The model under review builds one solid part; all positions refer to its coordinate system, in mm. Face numbers are marked on the shaded views. A direction names the side the tool comes from. Round coordinates to 2 decimals unless told otherwise and drop trailing zeros. Order: outer loops, then holes, each group sorted by start corner. A loop starts at its lowest first (then second) coordinate and runs counter-clockwise, first axis right, second up.
1) Clearance check with flat-ended pins moving along their axes: P1, Ø4, axis at y = 148.5, z = 55.5, coming from the -X side; P2, Ø9.5, axis at x = 0, y = 0, coming from the -Z side; P3, Ø3, axis at x = -1.5, y = -15, coming from the -Z side. State where each tip first meets the part, or that it passes through.
2) Mouldability with a two-part tool opening along Z and no side actions: class the marked faces 6, 7 and 8 as pulls with the +Z half, pulls with the -Z half, needs draft (parallel to the pull), parting line crosses it, or undercut.
3) Consider section B-B (y = 62.5). Give the boundary of the cut face in (x, z), then the cut area to 3 significant figures.
4) Machinability: for the marked faces 1, 2, 3, 4 and 5, which of the approach directions +Z, -Z, +X, -X, +Y, -Y give a long, thin tool a straight path to every point of the face, cutting with its end or side? Answer none if there is none.
5) To check wall thickness, follow L1, parallel to Y at x = 0, z = 11.25; L2, parallel to Z at x = 27, y = -24; L3, parallel to Y at x = 0, z = 4.75 (3 decimals). State the ranges of each line that lie inside material, in increasing order.
6) Consider section C-C (z = 203.5). Give the boundary of the cut face in (x, y), then the cut area to 3 significant figures.
7) Consider section A-A (z = 30.5). Give the boundary of the cut face in (x, y), then the cut area to 3 significant figures.
from build123d import *

# Parameters (mm, degrees)
SKETCH1_R            = 28.1
BOSS_EXTRUDE2_DEPTH  = 24
CUT_EXTRUDE2_DEPTH   = 21.5
SKETCH4_R            = 3
CUT_EXTRUDE3_DEPTH   = 9.5
SKETCH6_R            = 6.025
CUT_EXTRUDE4_DEPTH   = 6.2
SKETCH7_W            = 56.2
SKETCH7_H            = 56.2
BOSS_EXTRUDE3_DEPTH  = 56.2
SKETCH8_W            = 56.2
SKETCH8_H            = 56.2
BOSS_EXTRUDE4_DEPTH  = 14.14
SKETCH10_W           = 56.2
SKETCH10_H           = 56.2
BOSS_EXTRUDE5_DEPTH  = 10
SKETCH11_W           = 10
SKETCH11_H           = 56.2
BOSS_EXTRUDE6_DEPTH  = 146.9
SKETCH12_W           = 10
SKETCH12_H           = 56.2
BOSS_EXTRUDE7_DEPTH  = 126.9
SKETCH13_W           = 10
SKETCH13_H           = 56.2
BOSS_EXTRUDE8_DEPTH  = 146.9
SKETCH14_W           = 10
SKETCH14_H           = 56.2
BOSS_EXTRUDE9_DEPTH  = 126.9
SKETCH15_W           = 10
SKETCH15_H           = 56.2
BOSS_EXTRUDE10_DEPTH = 25
SKETCH16_W           = 10
SKETCH16_H           = 56.2
BOSS_EXTRUDE11_DEPTH = 25
SKETCH17_W           = 56.2
SKETCH17_H           = 10
BOSS_EXTRUDE12_DEPTH = 25
SKETCH18_W           = 56.2
SKETCH18_H           = 10
BOSS_EXTRUDE13_DEPTH = 25
SKETCH19_W           = 51.2
SKETCH19_H           = 51.2
CUT_EXTRUDE5_DEPTH   = 63.7
SKETCH23_W           = 330
SKETCH23_H           = 16.2
CUT_EXTRUDE7_DEPTH   = 5
SKETCH24_W           = 16.2
SKETCH24_H           = 290
CUT_EXTRUDE8_DEPTH   = 5
SKETCH25_W           = 16.2
SKETCH25_H           = 16.2
CUT_EXTRUDE12_DEPTH  = 25
CUT_EXTRUDE13_DEPTH  = 56.2
CUT_EXTRUDE14_DEPTH  = 56.2
SKETCH28_W           = 21
SKETCH28_H           = 16.2
CUT_EXTRUDE15_DEPTH  = 5
SKETCH29_W           = 21
SKETCH29_H           = 16.2
CUT_EXTRUDE16_DEPTH  = 5
SKETCH30_W           = 21
SKETCH30_H           = 16.2
CUT_EXTRUDE17_DEPTH  = 5
SKETCH31_W           = 21
SKETCH31_H           = 16.2
CUT_EXTRUDE18_DEPTH  = 5
SKETCH33_R           = 2.65
CUT_EXTRUDE19_DEPTH  = 2.4
SKETCH34_R           = 0.5
CUT_EXTRUDE20_DEPTH  = 10
SKETCH35_R           = 2.65
CUT_EXTRUDE21_DEPTH  = 2.4
SKETCH36_R           = 0.5
CUT_EXTRUDE22_DEPTH  = 10
SKETCH37_R           = 2.65
CUT_EXTRUDE23_DEPTH  = 2.4
SKETCH38_R           = 0.5
CUT_EXTRUDE24_DEPTH  = 10
SKETCH39_R           = 2.65
CUT_EXTRUDE25_DEPTH  = 2.4
SKETCH40_R           = 0.5
CUT_EXTRUDE26_DEPTH  = 10
SKETCH41_R           = 3.75
CUT_EXTRUDE28_DEPTH  = 30


with BuildPart() as part:
    # Sketch1 → Boss-Extrude2 (new body)
    with BuildSketch(Plane.XY):
        Circle(SKETCH1_R)
    extrude(amount=BOSS_EXTRUDE2_DEPTH)

    # Sketch3 → Cut-Extrude2 (cut)
    with BuildSketch(Plane(origin=(0, 0, 0), x_dir=(-1, 0, 0), z_dir=(0, 0, -1))):
        with BuildLine():
            Line((-1.661801922, 2.5), (1.661801922, 2.5))
            ThreePointArc((1.661801922, 2.5), (0, -3.001930317), (-1.661801922, 2.5))
        make_face()
    extrude(amount=-CUT_EXTRUDE2_DEPTH, mode=Mode.SUBTRACT)

    # Sketch4 → Cut-Extrude3 (cut)
    with BuildSketch(Plane(origin=(0, 0, 0), x_dir=(-1, 0, 0), z_dir=(0, 0, -1))):
        Circle(SKETCH4_R)
    extrude(amount=-CUT_EXTRUDE3_DEPTH, mode=Mode.SUBTRACT)

    # Sketch6 → Cut-Extrude4 (cut)
    with BuildSketch(Plane(origin=(0, 0, 0), x_dir=(-1, 0, 0), z_dir=(0, 0, -1))):
        Circle(SKETCH6_R)
    extrude(amount=-CUT_EXTRUDE4_DEPTH, mode=Mode.SUBTRACT)

    # Sketch7 → Boss-Extrude3 (add)
    with BuildSketch(Plane.XY.offset(24)):
        Rectangle(SKETCH7_W, SKETCH7_H)
    extrude(amount=BOSS_EXTRUDE3_DEPTH)

    # Sketch8 → Boss-Extrude4 (add)
    with BuildSketch(Plane(origin=(28.1, 0, 0), x_dir=(0, 0, -1), z_dir=(1, 0, 0))):
        with Locations((-52.1, 0)):
            Rectangle(SKETCH8_W, SKETCH8_H)
    extrude(amount=BOSS_EXTRUDE4_DEPTH)

    # Sketch10 → Boss-Extrude5 (add)
    with BuildSketch(Plane(origin=(42.24, 0, 0), x_dir=(0, 0, -1), z_dir=(1, 0, 0))):
        with Locations((-52.1, 0)):
            Rectangle(SKETCH10_W, SKETCH10_H)
    extrude(amount=BOSS_EXTRUDE5_DEPTH)

    # Sketch11 → Boss-Extrude6 (add)
    with BuildSketch(Plane.XY.offset(80.2)):
        with Locations((47.24, 0)):
            Rectangle(SKETCH11_W, SKETCH11_H)
    extrude(amount=BOSS_EXTRUDE6_DEPTH)

    # Sketch12 → Boss-Extrude7 (add)
    with BuildSketch(Plane(origin=(0, 28.1, 0), x_dir=(1, 0, 0), z_dir=(0, 1, 0))):
        with Locations((47.24, -52.1)):
            Rectangle(SKETCH12_W, SKETCH12_H)
    extrude(amount=BOSS_EXTRUDE7_DEPTH)

    # Sketch13 → Boss-Extrude8 (add)
    with BuildSketch(Plane(origin=(0, 0, 24), x_dir=(-1, 0, 0), z_dir=(0, 0, -1))):
        with Locations((-47.24, 0)):
            Rectangle(SKETCH13_W, SKETCH13_H)
    extrude(amount=BOSS_EXTRUDE8_DEPTH)

    # Sketch14 → Boss-Extrude9 (add)
    with BuildSketch(Plane(origin=(0, -28.1, 0), x_dir=(-1, 0, 0), z_dir=(0, -1, 0))):
        with Locations((-47.24, -52.1)):
            Rectangle(SKETCH14_W, SKETCH14_H)
    extrude(amount=BOSS_EXTRUDE9_DEPTH)

    # Sketch15 → Boss-Extrude10 (add)
    with BuildSketch(Plane(origin=(52.24, 0, 0), x_dir=(0, 0, -1), z_dir=(1, 0, 0))):
        with Locations((-222.1, 0)):
            Rectangle(SKETCH15_W, SKETCH15_H)
    extrude(amount=BOSS_EXTRUDE10_DEPTH)

    # Sketch16 → Boss-Extrude11 (add)
    with BuildSketch(Plane(origin=(52.24, 0, 0), x_dir=(0, 0, -1), z_dir=(1, 0, 0))):
        with Locations((117.9, 0)):
            Rectangle(SKETCH16_W, SKETCH16_H)
    extrude(amount=BOSS_EXTRUDE11_DEPTH)

    # Sketch17 → Boss-Extrude12 (add)
    with BuildSketch(Plane(origin=(52.24, 0, 0), x_dir=(0, 0, -1), z_dir=(1, 0, 0))):
        with Locations((-52.1, 150)):
            Rectangle(SKETCH17_W, SKETCH17_H)
    extrude(amount=BOSS_EXTRUDE12_DEPTH)

    # Sketch18 → Boss-Extrude13 (add)
    with BuildSketch(Plane(origin=(52.24, 0, 0), x_dir=(0, 0, -1), z_dir=(1, 0, 0))):
        with Locations((-52.1, -150)):
            Rectangle(SKETCH18_W, SKETCH18_H)
    extrude(amount=BOSS_EXTRUDE13_DEPTH)

    # Sketch19 → Cut-Extrude5 (cut)
    with BuildSketch(Plane.ZY.offset(28.1)):
        with Locations((52.1, 0)):
            Rectangle(SKETCH19_W, SKETCH19_H)
    extrude(amount=-CUT_EXTRUDE5_DEPTH, mode=Mode.SUBTRACT)

    # Cut-Sweep2: sweep along a path in Sketch20
    with BuildLine(Plane(origin=(0, 0, 0), x_dir=(-1, 0, 0), z_dir=(0, 0, -1))) as cut_sweep2_path:
        ThreePointArc((0, 15), (-10.606601718, 10.606601718), (-15, 0))
    # 3DSketch2 → Cut-Sweep2 (sweep, cut)
    with BuildSketch(Plane(origin=(0, 15, 0), x_dir=(0, 0.17521220324553322, 0.9845306921746249), z_dir=(-1, 0, 0))):
        Polygon((0, 0), (1.314091524, 7.383980191), (42.805237655, 0), (41.491146131, -7.383980191), align=None)
    sweep(path=cut_sweep2_path.line, mode=Mode.SUBTRACT)

    # Sketch23 → Cut-Extrude7 (cut)
    with BuildSketch(Plane(origin=(52.24, 0, 0), x_dir=(0, 0, -1), z_dir=(1, 0, 0))):
        with Locations((-52.1, 0)):
            Rectangle(SKETCH23_W, SKETCH23_H)
    extrude(amount=-CUT_EXTRUDE7_DEPTH, mode=Mode.SUBTRACT)

    # Sketch24 → Cut-Extrude8 (cut)
    with BuildSketch(Plane(origin=(52.24, 0, 0), x_dir=(0, 0, -1), z_dir=(1, 0, 0))):
        with Locations((-52.1, 0)):
            Rectangle(SKETCH24_W, SKETCH24_H)
    extrude(amount=-CUT_EXTRUDE8_DEPTH, mode=Mode.SUBTRACT)

    # Sketch25 → Cut-Extrude12 (cut)
    with BuildSketch(Plane(origin=(47.24, 0, 0), x_dir=(0, 0, -1), z_dir=(1, 0, 0))):
        with Locations((-52.1, 0)):
            Rectangle(SKETCH25_W, SKETCH25_H)
    extrude(amount=-CUT_EXTRUDE12_DEPTH, mode=Mode.SUBTRACT)

    # Sketch26 → Cut-Extrude13 (cut)
    with BuildSketch(Plane(origin=(0, -28.1, 0), x_dir=(-1, 0, 0), z_dir=(0, -1, 0))):
        Polygon((-77.24, -217.1), (-67.24, -227.1), (-77.24, -227.1), align=None)
        Polygon((-77.24, 112.9), (-67.24, 122.9), (-77.24, 122.9), align=None)
    extrude(amount=-CUT_EXTRUDE13_DEPTH, mode=Mode.SUBTRACT)

    # Sketch27 → Cut-Extrude14 (cut)
    with BuildSketch(Plane.XY.offset(80.2)):
        Polygon((77.24, -145), (67.24, -155), (77.24, -155), align=None)
        Polygon((77.24, 145), (67.24, 155), (77.24, 155), align=None)
    extrude(amount=-CUT_EXTRUDE14_DEPTH, mode=Mode.SUBTRACT)

    # Sketch28 → Cut-Extrude15 (cut)
    with BuildSketch(Plane(origin=(0, -145, 0), x_dir=(1, 0, 0), z_dir=(0, 1, 0))):
        with Locations((57.74, -52.1)):
            Rectangle(SKETCH28_W, SKETCH28_H)
    extrude(amount=-CUT_EXTRUDE15_DEPTH, mode=Mode.SUBTRACT)

    # Sketch29 → Cut-Extrude16 (cut)
    with BuildSketch(Plane(origin=(0, 145, 0), x_dir=(-1, 0, 0), z_dir=(0, -1, 0))):
        with Locations((-57.74, -52.1)):
            Rectangle(SKETCH29_W, SKETCH29_H)
    extrude(amount=-CUT_EXTRUDE16_DEPTH, mode=Mode.SUBTRACT)

    # Sketch30 → Cut-Extrude17 (cut)
    with BuildSketch(Plane(origin=(0, 0, 217.1), x_dir=(-1, 0, 0), z_dir=(0, 0, -1))):
        with Locations((-57.74, 0)):
            Rectangle(SKETCH30_W, SKETCH30_H)
    extrude(amount=-CUT_EXTRUDE17_DEPTH, mode=Mode.SUBTRACT)

    # Sketch31 → Cut-Extrude18 (cut)
    with BuildSketch(Plane.XY.offset(-112.9)):
        with Locations((57.74, 0)):
            Rectangle(SKETCH31_W, SKETCH31_H)
    extrude(amount=-CUT_EXTRUDE18_DEPTH, mode=Mode.SUBTRACT)

    # Sketch33 → Cut-Extrude19 (cut)
    with BuildSketch(Plane(origin=(147.17, 0, 147.17), x_dir=(0.7071067811865558, 0, -0.7071067811865392), z_dir=(0.7071067811865392, 0, 0.7071067811865558))):
        with Locations((-105.967022229, 4.05)):
            Circle(SKETCH33_R)
        with Locations((-105.967022229, -4.05)):
            Circle(SKETCH33_R)
    extrude(amount=-CUT_EXTRUDE19_DEPTH, mode=Mode.SUBTRACT)

    # Sketch34 → Cut-Extrude20 (cut)
    with BuildSketch(Plane(origin=(145.472943725, 0, 145.472943725), x_dir=(0.7071067811865559, 0, -0.7071067811865392), z_dir=(0.7071067811865392, 0, 0.7071067811865559))):
        with Locations((-105.967022229, 5.75)):
            Circle(SKETCH34_R)
        with Locations((-105.967022229, 2.35)):
            Circle(SKETCH34_R)
        with Locations((-105.967022229, -2.35)):
            Circle(SKETCH34_R)
        with Locations((-105.967022229, -5.75)):
            Circle(SKETCH34_R)
    extrude(amount=-CUT_EXTRUDE20_DEPTH, mode=Mode.SUBTRACT)

    # Sketch35 → Cut-Extrude21 (cut)
    with BuildSketch(Plane(origin=(95.07, 0, -95.07), x_dir=(-0.7071067811865392, 0, -0.7071067811865559), z_dir=(0.7071067811865559, 0, -0.7071067811865392))):
        with Locations((32.286495629, -4.05)):
            Circle(SKETCH35_R)
        with Locations((32.286495629, 4.05)):
            Circle(SKETCH35_R)
    extrude(amount=-CUT_EXTRUDE21_DEPTH, mode=Mode.SUBTRACT)

    # Sketch36 → Cut-Extrude22 (cut)
    with BuildSketch(Plane(origin=(93.372943725, 0, -93.372943725), x_dir=(-0.7071067811865392, 0, -0.7071067811865558), z_dir=(0.7071067811865558, 0, -0.7071067811865392))):
        with Locations((32.286495629, -5.75)):
            Circle(SKETCH36_R)
        with Locations((32.286495629, -2.35)):
            Circle(SKETCH36_R)
        with Locations((32.286495629, 2.35)):
            Circle(SKETCH36_R)
        with Locations((32.286495629, 5.75)):
            Circle(SKETCH36_R)
    extrude(amount=-CUT_EXTRUDE22_DEPTH, mode=Mode.SUBTRACT)

    # Sketch37 → Cut-Extrude23 (cut)
    with BuildSketch(Plane(origin=(111.12, -111.12, 0), x_dir=(0, 0, -1), z_dir=(0.707106781186554, -0.7071067811865411, 0))):
        with Locations(Location((-56.15, -54.984623305, 0), (0, 0, 90))):
            Circle(SKETCH37_R)
        with Locations(Location((-48.05, -54.984623305, 0), (0, 0, 90))):
            Circle(SKETCH37_R)
    extrude(amount=-CUT_EXTRUDE23_DEPTH, mode=Mode.SUBTRACT)

    # Sketch38 → Cut-Extrude24 (cut)
    with BuildSketch(Plane(origin=(109.422943725, -109.422943725, 0), x_dir=(0, 0, -1), z_dir=(0.7071067811865539, -0.7071067811865411, 0))):
        with Locations(Location((-57.85, -54.984623305, 0), (0, 0, 90))):
            Circle(SKETCH38_R)
        with Locations(Location((-54.45, -54.984623305, 0), (0, 0, 90))):
            Circle(SKETCH38_R)
        with Locations(Location((-49.75, -54.984623305, 0), (0, 0, 90))):
            Circle(SKETCH38_R)
        with Locations(Location((-46.35, -54.984623305, 0), (0, 0, 90))):
            Circle(SKETCH38_R)
    extrude(amount=-CUT_EXTRUDE24_DEPTH, mode=Mode.SUBTRACT)

    # Sketch39 → Cut-Extrude25 (cut)
    with BuildSketch(Plane(origin=(111.12, 111.12, 0), x_dir=(0.707106781186554, -0.7071067811865411, 0), z_dir=(0.7071067811865411, 0.707106781186554, 0))):
        with Locations(Location((-54.984623305, -48.05, 0), (0, 0, 180))):
            Circle(SKETCH39_R)
        with Locations(Location((-54.984623305, -56.15, 0), (0, 0, 180))):
            Circle(SKETCH39_R)
    extrude(amount=-CUT_EXTRUDE25_DEPTH, mode=Mode.SUBTRACT)

    # Sketch40 → Cut-Extrude26 (cut)
    with BuildSketch(Plane(origin=(109.422943725, 109.422943725, 0), x_dir=(0.7071067811865539, -0.7071067811865411, 0), z_dir=(0.7071067811865411, 0.7071067811865539, 0))):
        with Locations(Location((-54.984623305, -46.35, 0), (0, 0, 180))):
            Circle(SKETCH40_R)
        with Locations(Location((-54.984623305, -49.75, 0), (0, 0, 180))):
            Circle(SKETCH40_R)
        with Locations(Location((-54.984623305, -54.45, 0), (0, 0, 180))):
            Circle(SKETCH40_R)
        with Locations(Location((-54.984623305, -57.85, 0), (0, 0, 180))):
            Circle(SKETCH40_R)
    extrude(amount=-CUT_EXTRUDE26_DEPTH, mode=Mode.SUBTRACT)

    # Sketch41 → Cut-Extrude28 (cut)
    with BuildSketch(Plane(origin=(0, 0, 0), x_dir=(-1, 0, 0), z_dir=(0, 0, -1))):
        with Locations((0, 18.75)):
            Circle(SKETCH41_R)
        with Locations((-18.75, 0)):
            Circle(SKETCH41_R)
    extrude(amount=-CUT_EXTRUDE28_DEPTH, mode=Mode.SUBTRACT)


solid = part.part
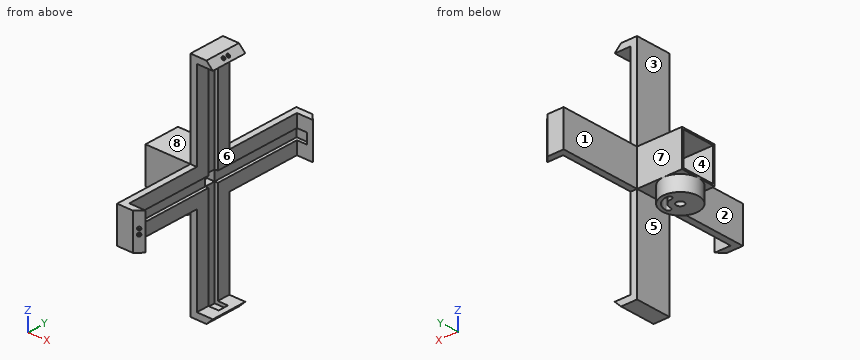
Answer below:
1. P1: stops at x = 42.24
1. P2: stops at z = 6.2
1. P3: stops at z = 0
2. face 6: undercut
2. face 7: needs draft
2. face 8: pulls with the +Z half
3. outline: (42.24, 24) - (52.24, 24) - (52.24, 44) - (47.24, 44) - (47.24, 60.2) - (52.24, 60.2) - (52.24, 80.2) - (42.24, 80.2) - close
3. area: 481 mm2
4. face 1: +Z, -Z, -X, +Y
4. face 2: +Z, -Z, -X, -Y
4. face 3: +Z, -X, +Y, -Y
4. face 4: -X
4. face 5: -Z, +Y, -Y
5. L1: y = -28.1 to -3, 2.5 to 15, 22.5 to 28.1
5. L2: z = 24 to 26.5, 77.7 to 80.2
5. L3: y = -28.1 to -6.025, 6.025 to 15, 22.5 to 28.1
6. outline: (42.24, -28.1) - (52.24, -28.1) - (52.24, -8.1) - (47.24, -8.1) - (47.24, 8.1) - (52.24, 8.1) - (52.24, 28.1) - (42.24, 28.1) - close
6. area: 481 mm2
7. outline: (-28.1, -28.1) - (42.24, -28.1) - (42.24, -155) - (67.24, -155) - (77.24, -145) - (52.24, -145) - (52.24, -8.1) - (47.24, -8.1) - (47.24, 8.1) - (52.24, 8.1) - (52.24, 145) - (77.24, 145) - (67.24, 155) - (42.24, 155) - (42.24, 28.1) - (-28.1, 28.1) - (-28.1, 25.6) - (35.6, 25.6) - (35.6, -25.6) - (-28.1, -25.6) - close
7. area: 4,110 mm2
